```python
from build123d import *

# Parameters (mm, degrees)
SKETCH1_W           = 128
SKETCH1_H           = 315
BOSS_EXTRUDE1_DEPTH = 3
SKETCH2_W           = 3
SKETCH2_H           = 312
SKETCH2_H_2         = 3
SKETCH2_W_2         = 122
BOSS_EXTRUDE3_DEPTH = 15


with BuildPart() as part:
    # Sketch1 → Boss-Extrude1 (new body)
    with BuildSketch(Plane.XY):
        Rectangle(SKETCH1_W, SKETCH1_H)
    extrude(amount=BOSS_EXTRUDE1_DEPTH)

    # Sketch2 → Boss-Extrude3 (add)
    with BuildSketch(Plane(origin=(0, 0, 0), x_dir=(-1, 0, 0), z_dir=(0, 0, -1))):
        with Locations((-62.5, 1.5)):
            Rectangle(SKETCH2_W, SKETCH2_H)
        with Locations((-62.5, -156)):
            Rectangle(SKETCH2_W, SKETCH2_H_2)
        with Locations((0, -156)):
            Rectangle(SKETCH2_W_2, SKETCH2_H_2)
        with Locations((62.5, 1.5)):
            Rectangle(SKETCH2_W, SKETCH2_H)
        with Locations((62.5, -156)):
            Rectangle(SKETCH2_W, SKETCH2_H_2)
    extrude(amount=BOSS_EXTRUDE3_DEPTH)


solid = part.part
```
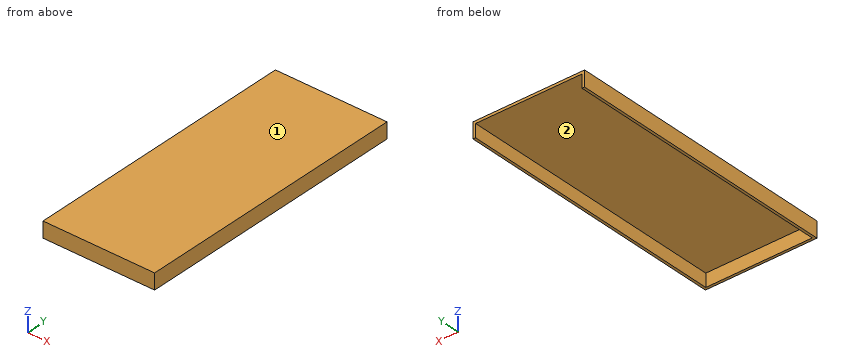
Source: CAD feature listing. Evaluate the final solid. Frame: model axes, mm. Face numbers are marked on the shaded views. A direction names the side the tool comes from. Round coordinates to 2 decimals unless told otherwise and drop trailing zeros. Loops run counter-clockwise (first coordinate to the right, second up) from the corner with the lowest first, then second, coordinate; pieces in that order, holes last. Notation, with made-up numbers: M 56,-11.75 L 71,-11.75 A20 cw 71,7.25 Z; hole C -10,31.25 d7. An arc over 180 degrees is marked long. Use a Markdown table: item, result. Add a question column.
1. Section query C-C on x = 38. Return the cut outline in (y, z), then the cut area to 3 significant figures.
2. Reachability of the marked faces 1 and 2 from +Z, -Z, +X, -X, +Y, -Y: full face, straight path, thin tool, end or side. Return the list, or none.
3. Section query A-A on y = -84.5. Return the cut outline in (x, z), then the cut area to 3 significant figures.
4. Contact query for a flat-ended pin moving along its axis: P1, Ø3, axis at x = -16.5, z = -2.5, coming from the +Y side. Output: stop coordinate, or through.
5. Line query: line 1 (X direction, y = -73, z = -12.75); line 2 (Z direction, x = -25.5, y = -104); line 3 (Y direction, x = 28.5, z = -1.75). Output: solid intervals per line, ascending.
6. Section query B-B on z = -5.25. Return the cut outline in (x, y).
Reported:
| question | item | result |
|---|---|---|
| 1 | outline | M -157.5,-15 L -154.5,-15 L -154.5,0 L 157.5,0 L 157.5,3 L -157.5,3 Z |
| 1 | area | 990 mm² |
| 2 | face 1 | +Z, +X, -X, +Y, -Y |
| 2 | face 2 | -Z, +Y |
| 3 | outline | M -64,-15 L -61,-15 L -61,0 L 61,0 L 61,-15 L 64,-15 L 64,3 L -64,3 Z |
| 3 | area | 474 mm² |
| 4 | P1 | stops at y = -154.5 |
| 5 | line 1 | x = -64 to -61, 61 to 64 |
| 5 | line 2 | z = 0 to 3 |
| 5 | line 3 | y = -157.5 to -154.5 |
| 6 | outline | M -64,-157.5 L 64,-157.5 L 64,157.5 L 61,157.5 L 61,-154.5 L -61,-154.5 L -61,157.5 L -64,157.5 Z |
